```python
from build123d import *

# Parameters (mm, degrees)
F1_DEPTH = 4
F2_T     = -1.5
F5_DEPTH = 2.5
F7_DEPTH = 4.001
F8_R     = 3
F9_R     = 1.5


# Not quite as in the source:
# - a feature names something its author has since deleted; it is built from what else it names


with BuildPart() as f1:
    # F0 (on Top) → F1 (new body)
    with BuildSketch(Plane.XY):
        with BuildLine():
            ThreePointArc((-6.5, 0), (-1.9038059223, 1.9038059223), (0, 6.5))
            Line((0, 6.5), (0, 47.4878030638))
            ThreePointArc((0, 47.4878030638), (-35.79631442, 35.8934680057), (-47.5090982427, 0.1357356025))
            Line((-47.5090982427, 0.1357356025), (-13, 0))
            Line((-13, 0), (-6.5, 0))
        make_face()
    extrude(amount=F1_DEPTH)

    # F2
    f2_openings = [f1.faces().sort_by_distance(p)[0] for p in [
        (-21.256566, 21.300379, 4),
        (-21.256566, 21.300379, 0),
    ]]
    offset(amount=F2_T, openings=f2_openings)

    # F4 (on offset) → F5 (join)
    with BuildSketch(Plane.XY.offset(2.5)):
        with BuildLine():
            Line((-46.2025064836, 1.6306079518), (-12.9970500154, 1.5))
            Line((-12.9970500154, 1.5), (-6.5, 1.5))
            ThreePointArc((-6.5, 1.5), (-2.9644660941, 2.9644660941), (-1.5, 6.5))
            Line((-1.5, 6.5), (-1.5, 46.186269666))
            ThreePointArc((-1.5, 46.186269666), (-34.737700628, 34.8307653134), (-46.2025064836, 1.6306079518))
        make_face()
    extrude(amount=-F5_DEPTH)

    # F6 (on face) → F7 (cut, through all)
    with BuildSketch(Plane.XY.offset(4)):
        with BuildLine():
            ThreePointArc((-1.5, 6.5), (-10.0355339059, 10.0355339059), (-6.5, 1.5))
            ThreePointArc((-6.5, 1.5), (-2.9644660941, 2.9644660941), (-1.5, 6.5))
        make_face()
    extrude(amount=-F7_DEPTH, mode=Mode.SUBTRACT)

    # F8
    f8_edges = [f1.edges().sort_by_distance(p)[0] for p in [
        (-47.509098, 0.135736, 2),
        (0, 47.487803, 2),
    ]]
    fillet(f8_edges, radius=F8_R)

    # F9
    f9_edges = [f1.edges().sort_by_distance(p)[0] for p in [
        (-46.202506, 1.630608, 3.25),
        (-1.5, 46.18627, 3.25),
    ]]
    fillet(f9_edges, radius=F9_R)


solid = f1.part
```
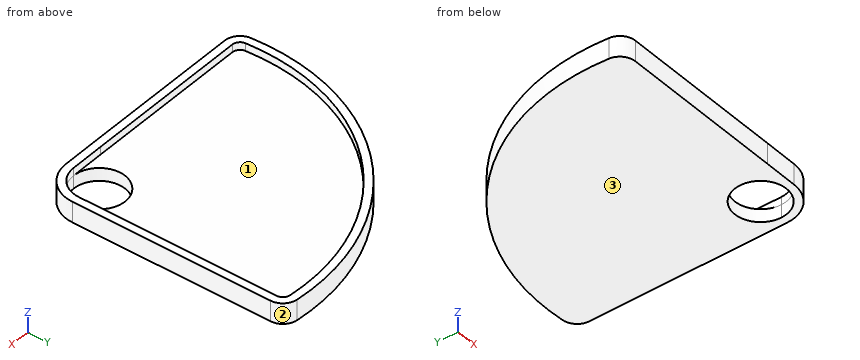
For this review, take the finished solid that the model builds, in its own axes (mm). Face numbers are marked on the shaded views. Round coordinates to 2 decimals unless told otherwise and drop trailing zeros. Write each loop counter-clockwise with the first axis right and the second up, starting at its lowest first coordinate (ties: lowest second). Pieces come first, ordered by that corner, then holes. Notation, with made-up numbers: (8, -13) - (32, -13) arc R29 ccw to (32, 21) - close; hole circle Ø6 at (75, 81). An arc over 180 degrees is marked (long way). Write each question's results on one line, items separated by ' | '.
Item 1: Draft analysis for pull direction X (two halves, no side actions). For the marked faces 1, 2 and 3, state which applies: pulls with the +X half, pulls with the -X half, needs draft (parallel to the pull), parting line crosses it, or undercut.
Calculated:
face 1: undercut | face 2: pulls with the +X half | face 3: needs draft
Item 2: Take a section at C-C on x = -14. State the section outline as (y, z) points.
Calculated:
outline: (0, 0) - (47.32, 0) - (47.32, 4) - (45.79, 4) - (45.79, 2.5) - (1.5, 2.5) - (1.5, 4) - (0, 4) - close
Item 3: Take a section at B-B on y = 5. State the section outline as (x, z) points.
Calculated:
outline: (-47.97, 0) - (-11.27, 0) - (-11.27, 2.5) - (-46.47, 2.5) - (-46.47, 4) - (-47.97, 4) - close; (-1.73, 0) - (-0.18, 0) - (-0.18, 4) - (-1.73, 4) - close
Item 4: Take a section at A-A on z = 1.1. State the section outline as (x, y) points, then the cut area to 3 significant figures.
Calculated:
outline: (-47.84, 2.86) arc R3 ccw to (-44.86, 0.13) - (-13, 0) - (-6.5, 0) arc R6.5 ccw to (0, 6.5) - (0, 44.84) arc R3 ccw to (-2.73, 47.83) arc R41.5 ccw to start; hole circle Ø10 at (-6.5, 6.5) | area: 1,840 mm^2
Item 5: To check wall thickness, follow line 1 along Y through (x, z) = (-6.5, 0.8); line 2 along X through (y, z) = (6.5, 2); line 3 along Z through (x, y) = (-10.5, 25). State the ranges of each line that lie inside material, in increasing order. Write a range as from..to.
Calculated:
line 1: y = 0..1.5, 11.5..48 | line 2: x = -48..-11.5, -1.5..0 | line 3: z = 0..2.5
Item 6: For pin 1 (13.5 mm diameter, centred on x = -16.5, y = 28, fed in from +Z); pin 2 (0.8 mm diameter, centred on x = -9, z = 3.5, fed in from +Y); pin 3 (1 mm diameter, centred on x = -25, z = 1.5, fed in from -Y), all flat-tipped, find the tip position at first contact; note any pin that passes through.
Calculated:
pin 1: stops at z = 2.5 | pin 2: stops at y = 47.95 | pin 3: stops at y = 0.05
Item 7: Take a section at D-D on y = 22.5. State the section outline as (x, z) points.
Calculated:
outline: (-44.79, 0) - (0, 0) - (0, 4) - (-1.5, 4) - (-1.5, 2.5) - (-43.16, 2.5) - (-43.16, 4) - (-44.79, 4) - close
